For this review, take the finished solid that the model builds, in its own axes (mm). A direction names the side the tool comes from. Round coordinates to 2 decimals unless told otherwise and drop trailing zeros. Order: outer loops, then holes, each group sorted by start corner. A loop starts at its lowest first (then second) coordinate and runs counter-clockwise, first axis right, second up. Notation, with made-up numbers: (31.5, -3.5) -> (88.5, -3.5) arc R10 ccw to (88.5, 0.5) -> close; hole circle Ø7 at (-21, -27.75). An arc over 180 degrees is marked (long way). Use a Markdown table: item, result. Add a question column.
1) Clearance check with flat-ended pins moving along their axes: P1, Ø10, axis at x = 3, y = 30.5, coming from the +Z side; P2, Ø3.5, axis at x = -4, z = -1.5, coming from the +Y side; P3, Ø1, axis at y = 23, z = 2.5, coming from the -X side. State where each tip first meets the part, or that it passes through.
2) Consider section C-C (y = 12). State the section outline as (x, z) points, plus the area to 3 significant figures.
3) Wall thickness on line 1 along Z through (x, y) = (0, 1.3); line 2 along Y through (x, z) = (-2.5, 5.75); line 3 along Z through (x, y) = (-0.5, 26): over which ranges is each line inside the solid? List them lowest first. Write a range as [from, to].
4) Consider section B-B (x = -5). State the section outline as (y, z) points.
5) Consider section A-A (z = 0). State the section outline as (x, y) points.
6) Draft analysis for pull direction X (two halves, no side actions). For faces 1 (the face through (-0.267, 2.465, 2.033)), 2 (the face through (0, 5, 0)), 3 (the face through (2.396, 36.378, -2.773)), 4 (the face through (-1.172, 8.381, -8.923)), state which applies: pulls with the +X half, pulls with the -X half, needs draft (parallel to the pull), parting line crosses it, or undercut.
7) Machinability: for faces 5 (the face through (2, 0, 2)), 6 (the face through (-4, 26, 0)), 7 (the face through (2, 17, 6)), which of the approach directions +Z, -Z, +X, -X, +Y, -Y give a long, thin tool a straight path to every point of the face, cutting with its end or side? Answer none if there is none.
8) Consider section D-D (z = -3.75). State the section outline as (x, y) points, plus the area to 3 significant figures.
```python
from build123d import *

# Parameters (mm, degrees)
SKETCH1_R           = 9
BOSS_EXTRUDE1_DEPTH = 17
SKETCH2_R           = 6
BOSS_EXTRUDE2_DEPTH = 9
CUT_EXTRUDE1_DEPTH  = 8.5
SKETCH4_R           = 2.25
BOSS_EXTRUDE3_DEPTH = 11
SKETCH5_R           = 2.25
SKETCH5_R_2         = 1.65
CUT_EXTRUDE2_DEPTH  = 4
SKETCH6_R           = 2.05
CUT_EXTRUDE3_DEPTH  = 5


with BuildPart() as part:
    # Sketch1 → Boss-Extrude1 (new body)
    with BuildSketch(Plane(origin=(0, 0, 0), x_dir=(1, 0, 0), z_dir=(0, 1, 0))):
        Circle(SKETCH1_R)
    extrude(amount=BOSS_EXTRUDE1_DEPTH)

    # Sketch2 → Boss-Extrude2 (add)
    with BuildSketch(Plane(origin=(0, 17, 0), x_dir=(1, 0, 0), z_dir=(0, 1, 0))):
        Circle(SKETCH2_R)
    extrude(amount=BOSS_EXTRUDE2_DEPTH)

    # Sketch3 → Cut-Extrude1 (cut, symmetric)
    with BuildSketch(Plane.XY):
        Polygon((-3, 26), (6, 26), (6, 24.8), align=None)
    extrude(amount=CUT_EXTRUDE1_DEPTH, both=True, mode=Mode.SUBTRACT)

    # Sketch4 → Boss-Extrude3 (add)
    with BuildSketch(Plane(origin=(3.35371179, 25.152838428, 0), x_dir=(0.991227901, -0.13216372, 0), z_dir=(0.13216372, 0.991227901, 0))):
        with Locations((-2.409940424, 2.75)):
            Circle(SKETCH4_R)
        with Locations((-2.409940424, -2.75)):
            Circle(SKETCH4_R)
    extrude(amount=BOSS_EXTRUDE3_DEPTH)

    # Sketch5 → Cut-Extrude2 (cut)
    with BuildSketch(Plane(origin=(4.807512711, 36.056345335, 0), x_dir=(0.991227901, -0.13216372, 0), z_dir=(0.13216372, 0.991227901, 0))):
        with Locations((-2.409940424, 2.75)):
            Circle(SKETCH5_R)
        with Locations((-2.409940424, 2.75)):
            Circle(SKETCH5_R_2, mode=Mode.SUBTRACT)
        with Locations((-2.409940424, -2.75)):
            Circle(SKETCH5_R)
        with Locations((-2.409940424, -2.75)):
            Circle(SKETCH5_R_2, mode=Mode.SUBTRACT)
    extrude(amount=-CUT_EXTRUDE2_DEPTH, mode=Mode.SUBTRACT)

    # Sketch6 → Cut-Extrude3 (cut)
    with BuildSketch(Plane.XZ):
        Circle(SKETCH6_R)
    extrude(amount=-CUT_EXTRUDE3_DEPTH, mode=Mode.SUBTRACT)


solid = part.part
```
Results list:
| question | item | result |
|---|---|---|
| 1 | P1 | z = 5 |
| 1 | P2 | y = 26 |
| 1 | P3 | x = -5.66 |
| 2 | outline | circle Ø18 at (0, 0) |
| 2 | area | 254 mm2 |
| 3 | line 1 | [-9, -2.05], [2.05, 9] |
| 3 | line 2 | [0, 17] |
| 3 | line 3 | [-4.41, -1.09], [1.09, 4.41] |
| 4 | outline | (0, -7.48) -> (17, -7.48) -> (17, -3.32) -> (26, -3.32) -> (26, 3.32) -> (17, 3.32) -> (17, 7.48) -> (0, 7.48) -> close |
| 5 | outline | (-9, 0) -> (-2.05, 0) -> (-2.05, 5) -> (2.05, 5) -> (2.05, 0) -> (9, 0) -> (9, 17) -> (6, 17) -> (6, 24.8) -> (-3, 26) -> (-6, 26) -> (-6, 17) -> (-9, 17) -> close |
| 6 | face 1 | undercut |
| 6 | face 2 | undercut |
| 6 | face 3 | pulls with the +X half |
| 6 | face 4 | parting line crosses it |
| 7 | face 5 | +Z, -Z, +X, -X, -Y |
| 7 | face 6 | +Z, -Z, -X, +Y |
| 7 | face 7 | +Y |
| 8 | outline | (-8.18, 0) -> (8.18, 0) -> (8.18, 17) -> (4.68, 17) -> (4.68, 24.98) -> (2.96, 25.2) -> (3.89, 32.14) -> (3.19, 32.24) -> (3.72, 36.2) -> (1.12, 36.55) -> (0.59, 32.58) -> (-0.11, 32.68) -> (-1.03, 25.74) -> (-3, 26) -> (-4.68, 26) -> (-4.68, 17) -> (-8.18, 17) -> close |
| 8 | area | 397 mm2 |
